Model file for the job. Use its own axes, mm. A direction names the side the tool comes from. Coordinates: 2 decimals unless noted, no trailing zeros. Write each loop counter-clockwise with the first axis right and the second up, starting at its lowest first coordinate (ties: lowest second). Pieces come first, ordered by that corner, then holes. Notation, with made-up numbers: (14.5, 26.25) -> (22.5, 26.25) arc R15 ccw to (22.5, 48.25) -> close; hole circle Ø5 at (9, 60.5). An arc over 180 degrees is marked (long way). Answer as a JSON object with one key per item and string values. Group by question number.
from build123d import *

# Parameters (mm, degrees)
SKETCH1_R           = 21
SKETCH1_R_2         = 1.75
SKETCH1_R_3         = 0.75
SKETCH1_R_4         = 7.5
BOSS_EXTRUDE1_DEPTH = 8
SKETCH2_R           = 3
CUT_EXTRUDE1_DEPTH  = 3


with BuildPart() as part:
    # Sketch1 → Boss-Extrude1 (new body)
    with BuildSketch(Plane(origin=(0, 0, 0), x_dir=(1, 0, 0), z_dir=(0, 1, 0))):
        with Locations(Location((0, 0, 0), (0, 0, 270))):
            Circle(SKETCH1_R)
        with Locations(Location((0, 15, 0), (0, 0, 270))):
            Circle(SKETCH1_R_2, mode=Mode.SUBTRACT)
        with Locations(Location((0, -15, 0), (0, 0, 270))):
            Circle(SKETCH1_R_3, mode=Mode.SUBTRACT)
        with Locations(Location((12.990381057, -7.5, 0), (0, 0, 270))):
            Circle(SKETCH1_R_2, mode=Mode.SUBTRACT)
        with Locations(Location((-12.990381057, -7.5, 0), (0, 0, 270))):
            Circle(SKETCH1_R_2, mode=Mode.SUBTRACT)
        with Locations(Location((-12.990381057, 7.5, 0), (0, 0, 270))):
            Circle(SKETCH1_R_3, mode=Mode.SUBTRACT)
        with Locations(Location((12.990381057, 7.5, 0), (0, 0, 270))):
            Circle(SKETCH1_R_3, mode=Mode.SUBTRACT)
        with Locations(Location((0, 0, 0), (0, 0, 270))):
            Circle(SKETCH1_R_4, mode=Mode.SUBTRACT)
    extrude(amount=BOSS_EXTRUDE1_DEPTH)

    # Sketch2 → Cut-Extrude1 (cut)
    with BuildSketch(Plane(origin=(0, 8, 0), x_dir=(1, 0, 0), z_dir=(0, 1, 0))):
        with Locations(Location((0, 15, 0), (0, 0, 270))):
            Circle(SKETCH2_R)
        with Locations(Location((12.990381057, -7.5, 0), (0, 0, 270))):
            Circle(SKETCH2_R)
        with Locations(Location((-12.990381057, -7.5, 0), (0, 0, 270))):
            Circle(SKETCH2_R)
    extrude(amount=-CUT_EXTRUDE1_DEPTH, mode=Mode.SUBTRACT)


solid = part.part
(1) Pin check, flat tips, straight feed: pin 1 (7 mm diameter, centred on x = 12.99, z = 7.5, fed in from -Y); pin 2 (5.5 mm diameter, centred on x = 12.99, z = 7.5, fed in from +Y); pin 3 (1.2 mm diameter, centred on x = 0, z = 15, fed in from +Y). Stop position of each tip, or through.
(2) Cut at A-A on x = 0. List the corners of the cut face in (y, z).
(3) Cut at D-D on z = 15. List the corners of the cut face in (x, y).
(4) Wall check: probe 1 along Z at (x, y) = (-1.5, 2.5); probe 2 along X at (y, z) = (0.75, 1); probe 3 along Y at (x, z) = (-14.5, 10). Give the ranges that are in metal, low to high.
(5) Cut at B-B on z = 0. List the corners of the cut face in (x, y).
(6) 3-axis set-ups, long thin cutter, end or side, ignore diameter. For faces 1 (the face through (12.258, 3.944, -7.663)), 2 (the face through (-15, 5, 7)): which of +Z, -Z, +X, -X, +Y, -Y reach the whole face in a straight line?
(7) Pull direction Z, two halves, no side cores. Call faces 3 (the face through (6.31, 3.94, 20.03)), 4 (the face through (-9, 8, 0)), 5 (the face through (14.466, 2.465, 8.441)): released by +Z, released by -Z, zero draft, split by the parting line, or undercut.
(8) Cut at C-C on y = 7.25. List the corners of the cut face in (x, z).
Results found:
{
 "1": {"pin 1": "stops at y = 0", "pin 2": "stops at y = 5", "pin 3": "passes through"},
 "2": {"outline": "(0, -21) -> (8, -21) -> (8, -18) -> (5, -18) -> (5, -16.75) -> (0, -16.75) -> close; (0, -13.25) -> (5, -13.25) -> (5, -12) -> (8, -12) -> (8, -7.5) -> (0, -7.5) -> close; (0, 7.5) -> (8, 7.5) -> (8, 14.25) -> (0, 14.25) -> close; (0, 15.75) -> (8, 15.75) -> (8, 21) -> (0, 21) -> close"},
 "3": {"outline": "(-14.7, 0) -> (-0.75, 0) -> (-0.75, 8) -> (-14.7, 8) -> close; (0.75, 0) -> (14.7, 0) -> (14.7, 8) -> (0.75, 8) -> close"},
 "4": {"probe 1": "z = -20.95 to -15.9, -14.1 to -7.35, 7.35 to 20.95", "probe 2": "x = -20.98 to -7.43, 7.43 to 20.98", "probe 3": "y = 0 to 5"},
 "5": {"outline": "(-21, 0) -> (-7.5, 0) -> (-7.5, 8) -> (-21, 8) -> close; (7.5, 0) -> (21, 0) -> (21, 8) -> (7.5, 8) -> close"},
 "6": {"face 1": "+Y, -Y", "face 2": "+Y"},
 "7": {"face 3": "split by the parting line", "face 4": "zero draft", "face 5": "undercut"},
 "8": {"outline": "circle Ø42 at (0, 0); hole circle Ø6 at (-12.99, 7.5); hole circle Ø1.5 at (-12.99, -7.5); hole circle Ø15 at (0, 0); hole circle Ø6 at (0, -15); hole circle Ø1.5 at (0, 15); hole circle Ø6 at (12.99, 7.5); hole circle Ø1.5 at (12.99, -7.5)"}
}
